Can you work these out from the model? Positions are in its coordinate system, mm. Face numbers are marked on the shaded views. A direction names the side the tool comes from. Round coordinates to 2 decimals unless told otherwise and drop trailing zeros. Order: outer loops, then holes, each group sorted by start corner. A loop starts at its lowest first (then second) coordinate and runs counter-clockwise, first axis right, second up. Notation, with made-up numbers: M 11,48.5 L 43,48.5 A29 ccw 43,81.5 Z; hole C 4.25,46.5 d3. An arc over 180 degrees is marked long. Answer as a JSON object with one key per item and string values. Group by question number.
from build123d import *

# Parameters (mm, degrees)
EXTRUDE1_DEPTH                 = 10
SKETCH2_W                      = 115
SKETCH2_H                      = 15
EXTRUDE2_DEPTH                 = 10
F_4_0_4_DIAMETER_HOLE1_D       = 4
F_4_0_4_DIAMETER_HOLE1_DEPTH   = 15
SKETCH4_W                      = 8
SKETCH4_H                      = 40
EXTRUDE3_DEPTH                 = 10
F_4_0_4_DIAMETER_HOLE3_D       = 4
F_4_0_4_DIAMETER_HOLE3_DEPTH   = 15
F_5_0_5_DIAMETER_HOLE1_D       = 5
F_5_0_5_DIAMETER_HOLE1_DEPTH   = 15
F_4_0_4_DIAMETER_HOLE5_D       = 4
F_4_0_4_DIAMETER_HOLE5_DEPTH   = 15
F_2_9_2_9_DIAMETER_HOLE1_D     = 2.9
F_2_9_2_9_DIAMETER_HOLE1_DEPTH = 10
SKETCH11_R                     = 9
EXTRUDE5_DEPTH                 = 10
SKETCH12_W                     = 45
SKETCH12_H                     = 25
EXTRUDE6_DEPTH                 = 10
SKETCH14_W                     = 20
SKETCH14_H                     = 25
EXTRUDE8_DEPTH                 = 5
F_4_0_4_DIAMETER_HOLE6_D       = 4
F_4_0_4_DIAMETER_HOLE6_DEPTH   = 15


with BuildPart() as part:
    # Sketch1 → Extrude1 (new body)
    with BuildSketch(Plane.XY):
        with BuildLine():
            Line((-65, -22.5), (65, -22.5))
            Line((65, -22.5), (65, 7.5))
            Line((65, 7.5), (63, 7.5))
            add(Edge.make_bspline(
                [(15, 22.5), (22.446642829, 21.197279562), (39.079741244, 18.287474734), (54.489303237, 11.338124296), (63, 7.5)],
                knots=[0, 0, 0, 0, 0.447700281, 1, 1, 1, 1], degree=3))
            Line((15, 22.5), (-15, 22.5))
            add(Edge.make_bspline(
                [(-15, 22.5), (-22.446642829, 21.197279562), (-39.079741244, 18.287474734), (-54.489303237, 11.338124296), (-63, 7.5)],
                knots=[0, 0, 0, 0, 0.447700281, 1, 1, 1, 1], degree=3))
            Line((-63, 7.5), (-65, 7.5))
            Line((-65, 7.5), (-65, -22.5))
        make_face()
    extrude(amount=EXTRUDE1_DEPTH)

    # Sketch2 → Extrude2 (add)
    with BuildSketch(Plane.XY):
        with Locations((0, -30)):
            Rectangle(SKETCH2_W, SKETCH2_H)
    extrude(amount=EXTRUDE2_DEPTH)

    # Ø4.0 (4) Diameter Hole1
    with Locations(Plane(origin=(-35, -31.5, 10), x_dir=(1, 0, 0), z_dir=(0, 0, 1))):
        with Locations((0, 0), (70, 0)):
            Hole(F_4_0_4_DIAMETER_HOLE1_D / 2, depth=F_4_0_4_DIAMETER_HOLE1_DEPTH)

    # Sketch4 → Extrude3 (add)
    with BuildSketch(Plane.XY.offset(10)):
        with Locations((0, -17.5)):
            Rectangle(SKETCH4_W, SKETCH4_H)
    extrude(amount=EXTRUDE3_DEPTH)

    # Ø4.0 (4) Diameter Hole3
    with Locations(Plane(origin=(25, 14.5, 0), x_dir=(-1, 0, 0), z_dir=(0, 0, -1))):
        with Locations((0, 0), (50, 0), (0, -8), (50, -8)):
            Hole(F_4_0_4_DIAMETER_HOLE3_D / 2, depth=F_4_0_4_DIAMETER_HOLE3_DEPTH)

    # Ø5.0 (5) Diameter Hole1
    with Locations(Plane(origin=(51.5, -31.5, 0), x_dir=(-1, 0, 0), z_dir=(0, 0, -1))):
        with Locations((0, 0)):
            f_5_0_5_diameter_hole1 = Hole(F_5_0_5_DIAMETER_HOLE1_D / 2, depth=F_5_0_5_DIAMETER_HOLE1_DEPTH)

    # Ø4.0 (4) Diameter Hole5
    with Locations(Plane(origin=(-8, -27.5, 10), x_dir=(1, 0, 0), z_dir=(0, 0, 1))):
        with Locations((0, 0), (16, 0), (8, 40)):
            Hole(F_4_0_4_DIAMETER_HOLE5_D / 2, depth=F_4_0_4_DIAMETER_HOLE5_DEPTH)

    # Mirror2: Ø5.0 (5) Diameter Hole1 across plane
    add(f_5_0_5_diameter_hole1.mirror(Plane(origin=(0, 0, 0), x_dir=(0, 0, 1), z_dir=(1, 0, 0))), mode=Mode.SUBTRACT)

    # Ø2.9 (2.9) Diameter Hole1
    with Locations(Plane(origin=(-4, -3.5, 15), x_dir=(0, -1, 0), z_dir=(-1, 0, 0))):
        with Locations((0, 0), (30, 0)):
            Hole(F_2_9_2_9_DIAMETER_HOLE1_D / 2, depth=F_2_9_2_9_DIAMETER_HOLE1_DEPTH)

    # Sketch11 → Extrude5 (cut)
    with BuildSketch(Plane.XY.offset(10)):
        with Locations((-17.597830753, -7.369190246)):
            Circle(SKETCH11_R)
    extrude5 = extrude(amount=-EXTRUDE5_DEPTH, mode=Mode.SUBTRACT)

    # Mirror3: Extrude5 across plane
    add(extrude5.mirror(Plane(origin=(0, 0, 0), x_dir=(0, 0, 1), z_dir=(1, 0, 0))), mode=Mode.SUBTRACT)

    # Sketch12 → Extrude6 (add)
    with BuildSketch(Plane.XY):
        with Locations((-87.5, -5)):
            Rectangle(SKETCH12_W, SKETCH12_H)
    extrude6 = extrude(amount=EXTRUDE6_DEPTH)

    # Sketch14 → Extrude8 (cut)
    with BuildSketch(Plane.XY.offset(10)):
        with Locations((-100, -5)):
            Rectangle(SKETCH14_W, SKETCH14_H)
    extrude8 = extrude(amount=-EXTRUDE8_DEPTH, mode=Mode.SUBTRACT)

    # Ø4.0 (4) Diameter Hole6
    with Locations(Plane(origin=(-104.2, 2.5, 5), x_dir=(1, 0, 0), z_dir=(0, 0, 1))):
        with Locations((0, 0), (0, -16)):
            f_4_0_4_diameter_hole6 = Hole(F_4_0_4_DIAMETER_HOLE6_D / 2, depth=F_4_0_4_DIAMETER_HOLE6_DEPTH)

    # Mirror5: Extrude6, Extrude8, Ø4.0 (4) Diameter Hole6 across plane
    add(extrude6.mirror(Plane(origin=(0, 0, 0), x_dir=(0, 0, 1), z_dir=(1, 0, 0))))
    add(extrude8.mirror(Plane(origin=(0, 0, 0), x_dir=(0, 0, 1), z_dir=(1, 0, 0))), mode=Mode.SUBTRACT)
    add(f_4_0_4_diameter_hole6.mirror(Plane(origin=(0, 0, 0), x_dir=(0, 0, 1), z_dir=(1, 0, 0))), mode=Mode.SUBTRACT)


solid = part.part
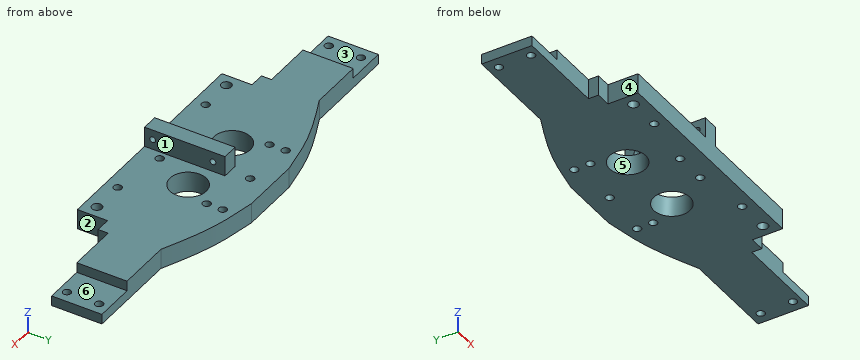
Item 1: Suppose I cut it at B-B, the plane x = -104.2. Write out the boundary of the cut face in (y, z).
Item 2: On a 3-axis mill with a long thin cutter (end or side, diameter ignored), from which of +Z, -Z, +X, -X, +Y, -Y can I reach the whole of each face in a straight line? I mean the marked faces 1, 2 and 3. Say none if no direction works.
Item 3: If we mould it in two halves opening along X, with no side actions, what happens to the marked faces 4, 5 and 6? For each: +X half, -X half, draft (parallel to the pull), parting line (faces both ways), or undercut.
Item 4: I need wall thicknesses on line 1 (X direction, y = -15, z = 6.5); line 2 (Z direction, x = -1, y = -33.5); line 3 (X direction, y = -12, z = 14.25). Which ranges of each line are inside material? Lowest first, please.
Item 5: I'm going to push flat-ended pins straight in: pin 1 Ø8 at (x, z) = (-70.5, 9) entering from -Y; pin 2 Ø3 at (x, z) = (-83.5, 4.5) entering from +Y; pin 3 Ø16 at (x, y) = (-97, -4) entering from +Z. Where does each tip first touch, or does it pass through?
Item 6: Suppose I cut it at A-A, the plane x = 0. Write out the boundary of the cut face in (y, z).
Computed:
{
 "1": {"outline": "M -17.5,0 L -15.5,0 L -15.5,5 L -17.5,5 Z; M -11.5,0 L 0.5,0 L 0.5,5 L -11.5,5 Z; M 4.5,0 L 7.5,0 L 7.5,5 L 4.5,5 Z"},
 "2": {"face 1": "+Z, +X, +Y, -Y", "face 2": "+Z, -Z, +X, -Y", "face 3": "+Z, -X, +Y, -Y"},
 "3": {"face 4": "-X half", "face 5": "undercut", "face 6": "draft"},
 "4": {"line 1": "x = -90 to -22.37, -12.83 to 12.83, 22.37 to 90", "line 2": "z = 0 to 13.55, 16.45 to 20", "line 3": "x = -4 to 4"},
 "5": {"pin 1": "stops at y = -17.5", "pin 2": "stops at y = 7.5", "pin 3": "stops at z = 10"},
 "6": {"outline": "M -37.5,0 L 10.5,0 L 10.5,10 L 2.5,10 L 2.5,20 L -37.5,20 Z; M 14.5,0 L 22.5,0 L 22.5,10 L 14.5,10 Z; hole C -33.5,15 d2.9; hole C -3.5,15 d2.9"}
}
